from build123d import *
from build123d.topology import SkipClean

# Parameters (mm, degrees)
ISO_START                                 = 20.256289073
ISO_SPUR_GEAR_0_8M_10T_20PA_8FW_2_R       = 0.4
ISO_SPUR_GEAR_0_8M_10T_20PA_8FW_S10_DEPTH = 8
BOSS_EXTRUDE1_DEPTH                       = 6
BOSS_EXTRUDE1_DEPTH_BACK                  = 8
SKETCH1_R                                 = 2.999
SKETCH2_R                                 = 2.4
CUT_EXTRUDE1_DEPTH                        = 3.2


# Read off the part's stored shape, not the designer's step: ISO - Spur gear 0.8M 10T 20PA 8FW ---S10A75H50L0.8N
with BuildPart() as part:
    # ISO - Spur gear 0.8M 10T 20PA 8FW -- 2 → ISO - Spur gear 0.8M 10T 20PA 8FW ---S10 (new body)
    with BuildSketch(Plane.YZ.offset(ISO_START)):
        with BuildLine():
            ThreePointArc((-8.829245422, -9.554744908), (-8.733282752, -9.555704257), (-8.637320082, -9.554744908))
            ThreePointArc((-8.637320082, -9.554744908), (-8.156276182, -8.696191622), (-8.268716011, -7.718503397))
            ThreePointArc((-8.268716011, -7.718503397), (-7.806540786, -7.60792275), (-7.367635501, -7.425724592))
            ThreePointArc((-7.367635501, -7.425724592), (-6.883930514, -8.282781454), (-5.990112863, -8.694615143))
            ThreePointArc((-5.990112863, -8.694615143), (-5.911913541, -8.63898583), (-5.834842001, -8.581804258))
            ThreePointArc((-5.834842001, -8.581804258), (-5.950314271, -7.604469549), (-6.615950723, -6.879593633))
            ThreePointArc((-6.615950723, -6.879593633), (-6.307040786, -6.518472229), (-6.059052342, -6.113088769))
            ThreePointArc((-6.059052342, -6.113088769), (-5.163961403, -6.522147678), (-4.198777965, -6.329955298))
            ThreePointArc((-4.198777965, -6.329955298), (-4.168211474, -6.23898583), (-4.139469773, -6.147423452))
            ThreePointArc((-4.139469773, -6.147423452), (-4.807351731, -5.42461596), (-5.771934306, -5.229430316))
            ThreePointArc((-5.771934306, -5.229430316), (-5.734282752, -4.755704258), (-5.771934306, -4.281978199))
            ThreePointArc((-5.771934306, -4.281978199), (-4.807351731, -4.086792554), (-4.139469773, -3.363985063))
            ThreePointArc((-4.139469773, -3.363985063), (-4.168211474, -3.272422685), (-4.198777965, -3.181453217))
            ThreePointArc((-4.198777965, -3.181453217), (-5.163961403, -2.989260837), (-6.059052342, -3.398319746))
            ThreePointArc((-6.059052342, -3.398319746), (-6.307040786, -2.992936286), (-6.615950723, -2.631814882))
            ThreePointArc((-6.615950723, -2.631814882), (-5.950314271, -1.906938966), (-5.834842001, -0.929604257))
            ThreePointArc((-5.834842001, -0.929604257), (-5.91191354, -0.872422684), (-5.990112863, -0.816793372))
            ThreePointArc((-5.990112863, -0.816793372), (-6.883930514, -1.228627061), (-7.367635501, -2.085683923))
            ThreePointArc((-7.367635501, -2.085683923), (-7.806540786, -1.903485765), (-8.268716011, -1.792905118))
            ThreePointArc((-8.268716011, -1.792905118), (-8.156276182, -0.815216893), (-8.637320082, 0.043336393))
            ThreePointArc((-8.637320082, 0.043336393), (-8.733282752, 0.044295743), (-8.829245422, 0.043336393))
            ThreePointArc((-8.829245422, 0.043336393), (-9.310289322, -0.815216893), (-9.197849493, -1.792905118))
            ThreePointArc((-9.197849493, -1.792905118), (-9.660024718, -1.903485765), (-10.098930003, -2.085683923))
            ThreePointArc((-10.098930003, -2.085683923), (-10.58263499, -1.228627061), (-11.476452641, -0.816793372))
            ThreePointArc((-11.476452641, -0.816793372), (-11.554651964, -0.872422684), (-11.631723503, -0.929604257))
            ThreePointArc((-11.631723503, -0.929604257), (-11.516251233, -1.906938966), (-10.850614781, -2.631814882))
            ThreePointArc((-10.850614781, -2.631814882), (-11.159524718, -2.992936286), (-11.407513162, -3.398319746))
            ThreePointArc((-11.407513162, -3.398319746), (-12.302604101, -2.989260837), (-13.267787539, -3.181453217))
            ThreePointArc((-13.267787539, -3.181453217), (-13.29835403, -3.272422685), (-13.327095731, -3.363985063))
            ThreePointArc((-13.327095731, -3.363985063), (-12.659213773, -4.086792554), (-11.694631199, -4.281978199))
            ThreePointArc((-11.694631199, -4.281978199), (-11.732282752, -4.755704258), (-11.694631199, -5.229430316))
            ThreePointArc((-11.694631199, -5.229430316), (-12.659213774, -5.42461596), (-13.327095731, -6.147423452))
            ThreePointArc((-13.327095731, -6.147423452), (-13.29835403, -6.23898583), (-13.267787539, -6.329955298))
            ThreePointArc((-13.267787539, -6.329955298), (-12.302604101, -6.522147678), (-11.407513162, -6.113088769))
            ThreePointArc((-11.407513162, -6.113088769), (-11.159524718, -6.518472229), (-10.850614781, -6.879593633))
            ThreePointArc((-10.850614781, -6.879593633), (-11.516251233, -7.604469549), (-11.631723503, -8.581804258))
            ThreePointArc((-11.631723503, -8.581804258), (-11.554651963, -8.63898583), (-11.476452641, -8.694615143))
            ThreePointArc((-11.476452641, -8.694615143), (-10.58263499, -8.282781454), (-10.098930003, -7.425724592))
            ThreePointArc((-10.098930003, -7.425724592), (-9.660024718, -7.60792275), (-9.197849493, -7.718503397))
            ThreePointArc((-9.197849493, -7.718503397), (-9.310289322, -8.696191622), (-8.829245422, -9.554744908))
        make_face()
        with Locations((-8.733282752, -4.755704257)):
            Circle(ISO_SPUR_GEAR_0_8M_10T_20PA_8FW_2_R, mode=Mode.SUBTRACT)
    extrude(amount=ISO_SPUR_GEAR_0_8M_10T_20PA_8FW_S10_DEPTH)

    # Sketch1 → Boss-Extrude1 (add, two sides: drawn at the far end of the back side and taken through both)
    with SkipClean():  # the faces are left unmerged after this step: merging them gives an invalid solid
        with BuildSketch(Plane.ZY.offset(-20.256289073).offset(-BOSS_EXTRUDE1_DEPTH_BACK)):
            with Locations((-4.755704257, -8.733282752)):
                Circle(SKETCH1_R)
        extrude(amount=BOSS_EXTRUDE1_DEPTH + BOSS_EXTRUDE1_DEPTH_BACK)

    # Sketch2 → Cut-Extrude1 (cut)
    with SkipClean():  # the faces are left unmerged after this step: merging them gives an invalid solid
        with BuildSketch(Plane.ZY.offset(-14.256289073)):
            with Locations((-4.755704257, -8.733282752)):
                Circle(SKETCH2_R)
        extrude(amount=-CUT_EXTRUDE1_DEPTH, mode=Mode.SUBTRACT)


solid = part.part
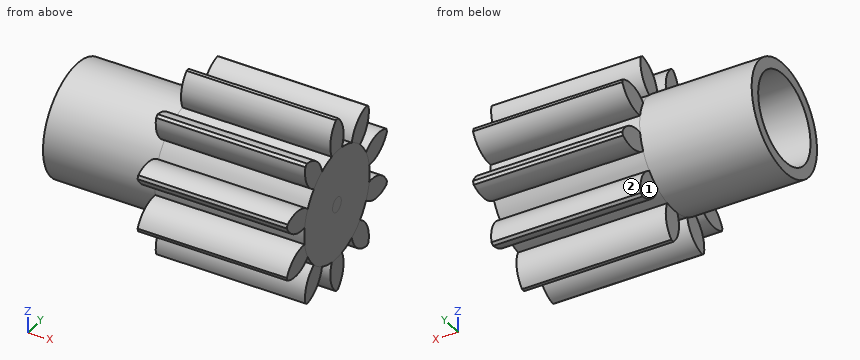
Model file for the job. Use its own axes, mm. Face numbers are marked on the shaded views. Give positions to 0.01 mm unless a question says otherwise; leave off trailing zeros. Order: outer loops, then holes, each group sorted by start corner. A loop starts at its lowest first (then second) coordinate and runs counter-clockwise, first axis right, second up. Notation, with made-up numbers: M 40,-14.5 L 68,-14.5 A13 cw 68,-9.5 Z; hole C 4,59 d5. An arc over 180 degrees is marked long. Put each result on its own line as item: value. Start each with the question number.
(1) Band-saw the part on D-D on x = 16.75. Give the cut face in (y, z), then the cut area to 3 significant figures.
(2) Drill centre lines: L1, parallel to Y at x = 23.5, z = -1; L2, parallel to Y at x = 25.25, z = -1.5; L3, parallel to X at y = -9.75, z = -4.75. Where is each one in solid material? Low to high. Write a range as [from, to].
(3) Pin check, flat tips, straight feed: pin 1 Ø1.4 at (y, z) = (-5, -5.5) entering from -X; pin 2 Ø4 at (y, z) = (-12, -3.5) entering from -X; pin 3 Ø1.5 at (x, y) = (18.5, -5.5) entering from -Z; pin 4 Ø2 at (x, z) = (23.5, -8) entering from -Y. Stop position of each tip, or through.
(4) Band-saw the part on C-C on y = -9.75. Give the cut face in (x, z).
(5) Band-saw the part on B-B on z = -1.25. Give the cut face in (x, y).
(6) Pull direction Z, two halves, no side cores. Call the marked faces 1 and 2: released by +Z, released by -Z, zero draft, split by the parting line, or undercut.
(7) Band-saw the part on A-A on y = -4.75. Give the cut face in (x, z), then the cut area to 3 significant figures.
Results below:
1. outline: C -8.73,-4.76 d6; hole C -8.73,-4.76 d4.8
1. area: 10.2 mm2
2. L1: y = [-11.64, -10.9], [-9.34, -8.13], [-6.56, -5.82]
2. L2: y = [-11.64, -10.35], [-9.3, -8.17], [-7.12, -5.83]
2. L3: x = [17.46, 28.26]
3. pin 1: stops at x = 20.26
3. pin 2: stops at x = 14.26
3. pin 3: stops at z = -6.44
3. pin 4: stops at y = -11.66
4. outline: M 14.26,-7.58 L 28.26,-7.58 L 28.26,-1.93 L 14.26,-1.93 L 14.26,-2.58 L 17.46,-2.58 L 17.46,-6.93 L 14.26,-6.93 Z
5. outline: M 20.26,-11.66 L 28.26,-11.66 L 28.26,-10.56 L 20.26,-10.56 Z; M 20.26,-9.34 L 28.26,-9.34 L 28.26,-8.13 L 20.26,-8.13 Z; M 20.26,-6.91 L 28.26,-6.91 L 28.26,-5.8 L 20.26,-5.8 Z
6. face 1: zero draft
6. face 2: undercut
7. outline: M 20.26,-6.52 L 28.26,-6.52 L 28.26,-5.46 L 20.26,-5.46 Z; M 20.26,-4.05 L 28.26,-4.05 L 28.26,-2.99 L 20.26,-2.99 Z
7. area: 16.9 mm2
